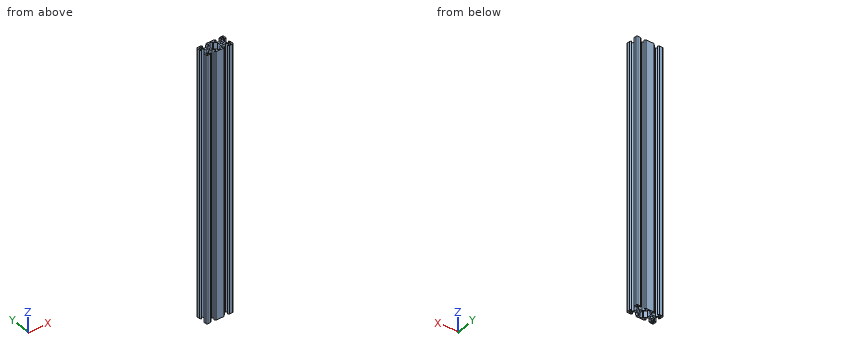
```python
from build123d import *

# Parameters (mm, degrees)
F1_DEPTH = 400


with BuildPart() as f1:
    # F0 (on Top) → F1 (new body)
    with BuildSketch(Plane.XY):
        with BuildLine():
            ThreePointArc((-43.014015, 11.811976), (-44.286807, 11.284768), (-44.814015, 10.011976))
            Line((-44.814015, 10.011976), (-44.814015, 6.001976))
            Line((-44.814015, 6.001976), (-43.014015, 4.201976))
            Line((-43.014015, 4.201976), (-43.014015, 7.041976))
            Line((-43.014015, 7.041976), (-41.294215, 7.041976))
            Line((-41.294215, 7.041976), (-38.746832, 4.651976))
            Line((-38.746832, 4.651976), (-38.746832, 1.811976))
            Line((-38.746832, 1.811976), (-38.746832, -1.028024))
            Line((-38.746832, -1.028024), (-41.294215, -3.418024))
            Line((-41.294215, -3.418024), (-43.014015, -3.418024))
            Line((-43.014015, -3.418024), (-43.014015, -0.578024))
            Line((-43.014015, -0.578024), (-44.814015, -2.378024))
            Line((-44.814015, -2.378024), (-44.814015, -6.388024))
            ThreePointArc((-44.814015, -6.388024), (-44.286807, -7.660816), (-43.014015, -8.188024))
            Line((-43.014015, -8.188024), (-39.004015, -8.188024))
            Line((-39.004015, -8.188024), (-37.204015, -6.388024))
            Line((-37.204015, -6.388024), (-40.304332, -6.388024))
            Line((-40.304332, -6.388024), (-40.304332, -4.488024))
            Line((-40.304332, -4.488024), (-37.652902, -2.120841))
            Line((-37.652902, -2.120841), (-34.814015, -2.120841))
            Line((-34.814015, -2.120841), (-31.975129, -2.120841))
            Line((-31.975129, -2.120841), (-29.323698, -4.488024))
            Line((-29.323698, -4.488024), (-29.323698, -6.388024))
            Line((-29.323698, -6.388024), (-32.424015, -6.388024))
            Line((-32.424015, -6.388024), (-30.624015, -8.188024))
            Line((-30.624015, -8.188024), (-26.614015, -8.188024))
            Line((-26.614015, -8.188024), (-23.014015, -8.188024))
            Line((-23.014015, -8.188024), (-19.004015, -8.188024))
            Line((-19.004015, -8.188024), (-17.204015, -6.388024))
            Line((-17.204015, -6.388024), (-20.304332, -6.388024))
            Line((-20.304332, -6.388024), (-20.304332, -4.488024))
            Line((-20.304332, -4.488024), (-17.652902, -2.120841))
            Line((-17.652902, -2.120841), (-14.814015, -2.120841))
            Line((-14.814015, -2.120841), (-11.975129, -2.120841))
            Line((-11.975129, -2.120841), (-9.323698, -4.488024))
            Line((-9.323698, -4.488024), (-9.323698, -6.388024))
            Line((-9.323698, -6.388024), (-12.424015, -6.388024))
            Line((-12.424015, -6.388024), (-10.624015, -8.188024))
            Line((-10.624015, -8.188024), (-6.614015, -8.188024))
            ThreePointArc((-6.614015, -8.188024), (-5.341223, -7.660816), (-4.814015, -6.388024))
            Line((-4.814015, -6.388024), (-4.814015, -2.378024))
            Line((-4.814015, -2.378024), (-6.614015, -0.578024))
            Line((-6.614015, -0.578024), (-6.614015, -3.418024))
            Line((-6.614015, -3.418024), (-8.333815, -3.418024))
            Line((-8.333815, -3.418024), (-10.881198, -1.028024))
            Line((-10.881198, -1.028024), (-10.881198, 1.811976))
            Line((-10.881198, 1.811976), (-10.881198, 4.651976))
            Line((-10.881198, 4.651976), (-8.333815, 7.041976))
            Line((-8.333815, 7.041976), (-6.614015, 7.041976))
            Line((-6.614015, 7.041976), (-6.614015, 4.201976))
            Line((-6.614015, 4.201976), (-4.814015, 6.001976))
            Line((-4.814015, 6.001976), (-4.814015, 10.011976))
            ThreePointArc((-4.814015, 10.011976), (-5.341223, 11.284768), (-6.614015, 11.811976))
            Line((-6.614015, 11.811976), (-10.624015, 11.811976))
            Line((-10.624015, 11.811976), (-12.424015, 10.011976))
            Line((-12.424015, 10.011976), (-9.323698, 10.011976))
            Line((-9.323698, 10.011976), (-9.323698, 8.111976))
            Line((-9.323698, 8.111976), (-11.975129, 5.744793))
            Line((-11.975129, 5.744793), (-14.814015, 5.744793))
            Line((-14.814015, 5.744793), (-17.652902, 5.744793))
            Line((-17.652902, 5.744793), (-20.304332, 8.111976))
            Line((-20.304332, 8.111976), (-20.304332, 10.011976))
            Line((-20.304332, 10.011976), (-17.204015, 10.011976))
            Line((-17.204015, 10.011976), (-19.004015, 11.811976))
            Line((-19.004015, 11.811976), (-23.014015, 11.811976))
            Line((-23.014015, 11.811976), (-26.614015, 11.811976))
            Line((-26.614015, 11.811976), (-30.624015, 11.811976))
            Line((-30.624015, 11.811976), (-32.424015, 10.011976))
            Line((-32.424015, 10.011976), (-29.323698, 10.011976))
            Line((-29.323698, 10.011976), (-29.323698, 8.111976))
            Line((-29.323698, 8.111976), (-31.975129, 5.744793))
            Line((-31.975129, 5.744793), (-34.814015, 5.744793))
            Line((-34.814015, 5.744793), (-37.652902, 5.744793))
            Line((-37.652902, 5.744793), (-40.304332, 8.111976))
            Line((-40.304332, 8.111976), (-40.304332, 10.011976))
            Line((-40.304332, 10.011976), (-37.204015, 10.011976))
            Line((-37.204015, 10.011976), (-39.004015, 11.811976))
            Line((-39.004015, 11.811976), (-43.014015, 11.811976))
        make_face()
        Polygon((-43.014015, -4.488024), (-42.434675, -4.488024), (-41.374332, -5.443314), (-41.374332, -6.388024), (-43.014015, -6.388024), align=None, mode=Mode.SUBTRACT)
        Polygon((-6.614015, -6.388024), (-8.253698, -6.388024), (-8.253698, -5.443314), (-7.193355, -4.488024), (-6.614015, -4.488024), align=None, mode=Mode.SUBTRACT)
        with BuildLine():
            ThreePointArc((-36.914015, 1.811976), (-36.298939, 3.2969), (-34.814015, 3.911976))
            ThreePointArc((-34.814015, 3.911976), (-33.329091, 3.2969), (-32.714015, 1.811976))
            ThreePointArc((-32.714015, 1.811976), (-33.329091, 0.327052), (-34.814015, -0.288024))
            ThreePointArc((-34.814015, -0.288024), (-36.298939, 0.327052), (-36.914015, 1.811976))
        make_face(mode=Mode.SUBTRACT)
        Polygon((-30.881198, 1.811976), (-30.881198, 4.651976), (-27.193355, 8.111976), (-27.193355, 10.011976), (-22.434675, 10.011976), (-22.434675, 8.111976), (-18.746832, 4.651976), (-18.746832, 1.811976), (-18.746832, -1.028024), (-22.434675, -4.488024), (-22.434675, -6.388024), (-27.193355, -6.388024), (-27.193355, -4.488024), (-30.881198, -1.028024), align=None, mode=Mode.SUBTRACT)
        Polygon((-43.014015, 8.111976), (-43.014015, 10.011976), (-41.374332, 10.011976), (-41.374332, 9.067266), (-42.434675, 8.111976), align=None, mode=Mode.SUBTRACT)
        with BuildLine():
            ThreePointArc((-16.914015, 1.811976), (-16.298939, 3.2969), (-14.814015, 3.911976))
            ThreePointArc((-14.814015, 3.911976), (-13.329091, 3.2969), (-12.714015, 1.811976))
            ThreePointArc((-12.714015, 1.811976), (-13.329091, 0.327052), (-14.814015, -0.288024))
            ThreePointArc((-14.814015, -0.288024), (-16.298939, 0.327052), (-16.914015, 1.811976))
        make_face(mode=Mode.SUBTRACT)
        Polygon((-8.253698, 9.067266), (-8.253698, 10.011976), (-6.614015, 10.011976), (-6.614015, 8.111976), (-7.193355, 8.111976), align=None, mode=Mode.SUBTRACT)
    extrude(amount=F1_DEPTH)


solid = f1.part
```
Verification items for the finished model (mm, model axes). Coordinates: 2 decimals unless noted, no trailing zeros. One line per question, with ' | ' between items. Start each with the question number.
1. Section check A-A (z = 239). Count the separate pieces of the cut face and the enclosed holes in it, plus the area to 3 significant figures.
2. Material ranges on line 1 along Y through (x, z) = (-7, 271); line 2 along X through (y, z) = (1.5, 328.5); line 3 along X through (y, z) = (-2, 328), recorded low to high.
3. Gauge pin test, flat ends, axial feed: P1, Ø4, axis at y = 1, z = 337.5, coming from the -X side; P2, Ø6, axis at x = -23.5, y = 9, coming from the +Z side; P3, Ø3, axis at x = -35.5, z = 84.5, coming from the -Y side; P4, Ø4.5, axis at x = -35.5, z = 132.5, coming from the -Y side. Record the tip position at first contact, or that the pin passes through.
Computed values:
1) separate pieces: 1 | enclosed holes: 7 | area: 303 mm²
2) line 1: -8.19 to -6.39, -4.49 to -3.42, 7.04 to 8.11, 10.01 to 11.81 | line 2: -38.75 to -36.89, -32.74 to -30.88, -18.75 to -16.89, -12.74 to -10.88 | line 3: -44.44 to -43.01, -39.78 to -29.85, -19.78 to -9.85, -6.61 to -5.19
3) P1: x = -43.44 | P2: z = 400 | P3: y = -2.12 | P4: y = -6.93
